from build123d import *

# Parameters (mm, degrees)
F0_W     = 150
F0_H     = 30
F0_W_2   = 10
F0_H_2   = 10
F1_DEPTH = 15
F2_SIZE  = 3


with BuildPart() as f1:
    # F0 (on Top) → F1 (new body)
    with BuildSketch(Plane.XY):
        with Locations((60, 0)):
            Rectangle(F0_W, F0_H)
        Rectangle(F0_W_2, F0_H_2, mode=Mode.SUBTRACT)
    extrude(amount=F1_DEPTH)

    # F2
    f2_edges = [f1.edges().sort_by_distance(p)[0] for p in [
        (60, -15, 15),
        (135, -15, 7.5),
        (60, -15, 0),
        (135, 0, 0),
        (135, 15, 7.5),
        (135, 0, 15),
        (60, 15, 15),
        (-15, 0, 15),
        (-15, -15, 7.5),
        (-15, 15, 7.5),
        (-15, 0, 0),
        (60, 15, 0),
    ]]
    chamfer(f2_edges, length=F2_SIZE)


solid = f1.part
For this review, take the finished solid that the model builds, in its own axes (mm). A direction names the side the tool comes from. Give positions to 0.01 mm unless a question says otherwise; leave off trailing zeros. Loops run counter-clockwise (first coordinate to the right, second up) from the corner with the lowest first, then second, coordinate; pieces in that order, holes last.
Item 1: Tool access review of faces 4 (the flat face through (59, 13, 1)), 5 (the flat face through (0, -5, 7)): name each direction out of +Z, -Z, +X, -X, +Y, -Y from which nothing blocks a thin tool from reaching the whole face with its end or side.
Item 2: Take a section at A-A, the plane z = 8. State the section outline as (x, y) points, and give its area (3 significant figures).
Item 3: Draft analysis for pull direction X (two halves, no side actions). For faces 1 (the flat face through (-5, 0, 7)), 2 (the flat face through (-13, 13, 2)), 3 (the flat face through (133, 0, 1)), state which applies: +X half, -X half, draft (parallel to the pull), parting line (faces both ways), or undercut.
Item 4: Take a section at B-B, the plane x = 2. State the section outline as (y, z) points, and give its area (3 significant figures).
Item 5: For line 1 along X through (y, z) = (4, 7.5); line 2 along Y through (x, z) = (1, 4.5); line 3 along X through (y, z) = (4, 13.25), list the stretches that pass through material, from the lowest coordinate up.
Item 6: Take a section at C-C, the plane x = 47.5. State the section outline as (y, z) points.
Calculated:
1. face 4: -Z, +X, -X, +Y
1. face 5: +Z, -Z
2. outline: (-15, -12) - (-12, -15) - (132, -15) - (135, -12) - (135, 12) - (132, 15) - (-12, 15) - (-15, 12) - close; hole (-5, -5) - (5, -5) - (5, 5) - (-5, 5) - close
2. area: 4,380 mm2
3. face 1: undercut
3. face 2: -X half
3. face 3: +X half
4. outline: (-15, 3) - (-12, 0) - (-5, 0) - (-5, 15) - (-12, 15) - (-15, 12) - close; (5, 0) - (12, 0) - (15, 3) - (15, 12) - (12, 15) - (5, 15) - close
4. area: 282 mm2
5. line 1: x = -15 to -5, 5 to 135
5. line 2: y = -15 to -5, 5 to 15
5. line 3: x = -13.75 to -5, 5 to 133.75
6. outline: (-15, 3) - (-12, 0) - (12, 0) - (15, 3) - (15, 12) - (12, 15) - (-12, 15) - (-15, 12) - close
